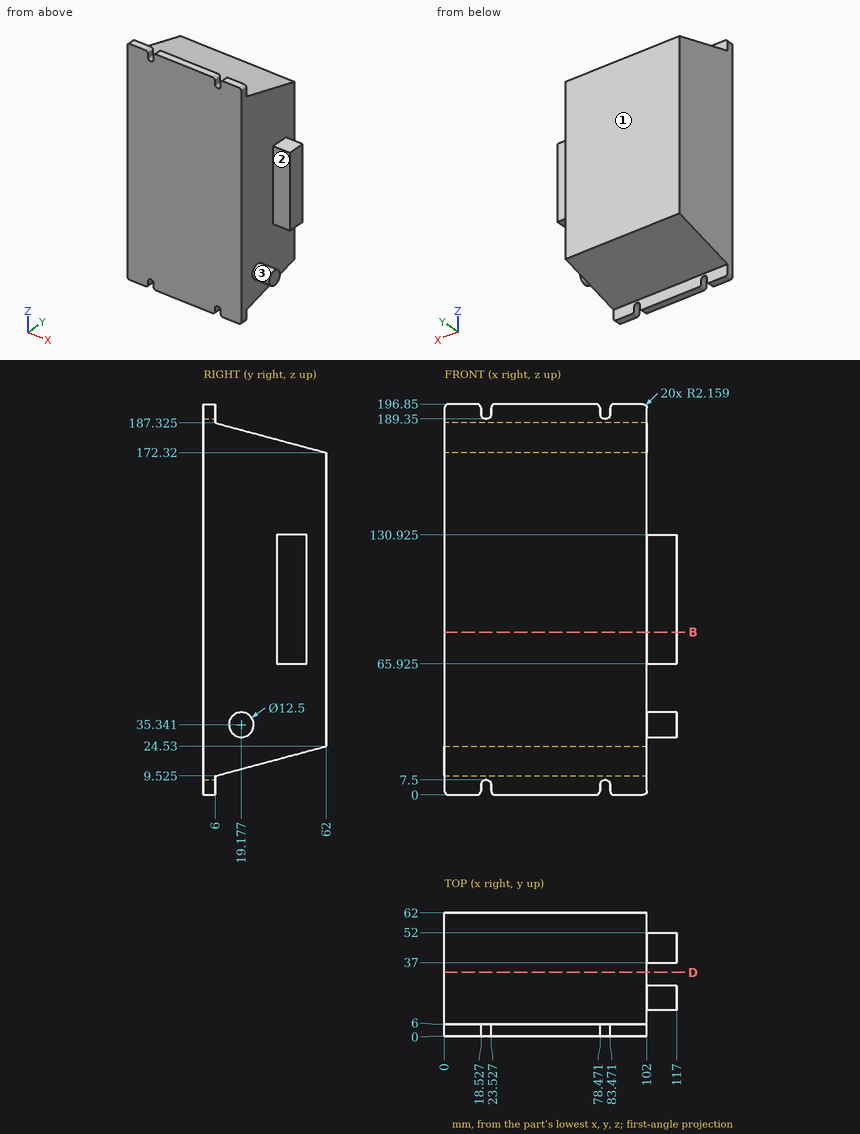
Verification items for this drawing (mm, ordinates from the low corner). A direction names the side the tool comes from. Round coordinates to 2 decimals unless told otherwise and drop trailing zeros. Order: outer loops, then holes, each group sorted by start corner. A loop starts at its lowest first (then second) coordinate and runs counter-clockwise, first axis right, second up. Notation, with made-up numbers: (60, 17.25) - (100, 17.25) arc R24 cw to (100, 46.25) - close; hole circle Ø11 at (80, 15). An arc over 180 degrees is marked (long way). Use CSV: the item, a comma, the result in double quotes.
(1) Section check D-D on y = 32. Record the boundary of the cut face in (x, z), and give its area (3 significant figures).
Entries:
outline,"(0, 16.49) - (102, 16.49) - (102, 180.36) - (0, 180.36) - close"
area,"16,700 mm^2"
(2) Gauge pin test, flat ends, axial feed: pin 1 Ø12 at (x, y) = (110.5, 41.5) entering from +Z (3 decimals); pin 2 Ø12 at (x, y) = (92, 30) entering from -Z; pin 3 Ø5 at (y, z) = (25.5, 171) entering from -X; pin 4 Ø1 at (y, z) = (4, 193) entering from +X. Record the tip position at first contact, or that the pin passes through.
Entries:
pin 1,"z = 130.925"
pin 2,"z = 14.35"
pin 3,"x = 0"
pin 4,"x = 102"
(3) Access from +Z, -Z, +X, -X, +Y, -Y to the whole of each face (thin tool, end or side, straight path). Record for the marked faces 1, 2 and 3.
Entries:
face 1,"+Z, -Z, +X, -X, +Y"
face 2,"+Z, -Z, +X, -Y"
face 3,"+X"
(4) Thickness scan on probe 1 along X at (y, z) = (31, 88.5); probe 2 along Z at (x, y) = (110, 45.5) (1 decimal); probe 3 along Z at (x, y) = (93, 46.5). Record the ranges inside material, lowest first. Write a range as from..to.
Entries:
probe 1,"0..102"
probe 2,"65.9..130.9"
probe 3,"20.38..176.47"
(5) Section check B-B on z = 82. Record the boundary of the cut face in (x, y).
Entries:
outline,"(0, 0) - (102, 0) - (102, 37) - (117, 37) - (117, 52) - (102, 52) - (102, 62) - (0, 62) - close"
